Geometry check sheet. Reference: the model listing, model coordinates, mm. Face numbers are marked on the shaded views. Give positions to 0.01 mm unless a question says otherwise; leave off trailing zeros. Order: outer loops, then holes, each group sorted by start corner. A loop starts at its lowest first (then second) coordinate and runs counter-clockwise, first axis right, second up. Notation, with made-up numbers: M -13,-1 L 0,-1 A15 cw 0,10 Z; hole C 80.5,45 d10. An arc over 180 degrees is marked long. Answer as CSV lines item,"result". Start each with the question number.
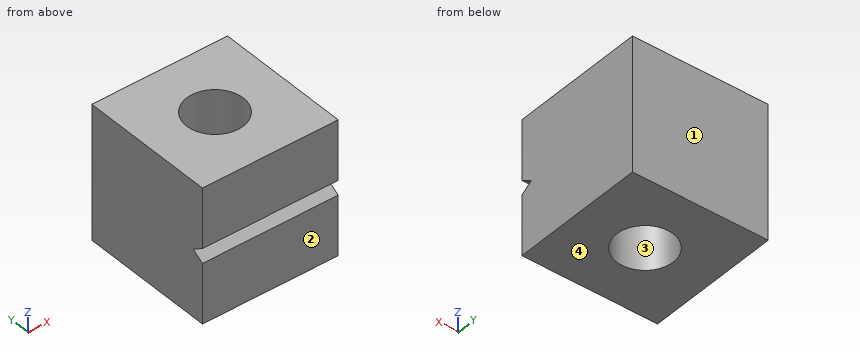
```python
from build123d import *

# Parameters (mm, degrees)
SKETCH1_W               = 19.05
SKETCH1_H               = 19.05
BOSS_EXTRUDE1_DEPTH     = 18.796
SKETCH2_R               = 3.9624
CUT_EXTRUDE1_DEPTH      = 24.124464664
CUT_EXTRUDE2_DEPTH      = 24.124464664
CUT_EXTRUDE2_DEPTH_BACK = 24.124464664


with BuildPart() as part:
    # Sketch1 → Boss-Extrude1 (new body)
    with BuildSketch(Plane.XY):
        Rectangle(SKETCH1_W, SKETCH1_H)
    extrude(amount=BOSS_EXTRUDE1_DEPTH)

    # Sketch2 → Cut-Extrude1 (cut, through all)
    with BuildSketch(Plane.XY.offset(18.796)):
        Circle(SKETCH2_R)
    extrude(amount=-CUT_EXTRUDE1_DEPTH, mode=Mode.SUBTRACT)

    # Sketch3 → Cut-Extrude2 (cut, two sides: drawn at the far end of the back side and taken through both)
    with BuildSketch(Plane(origin=(0, 0, 0), x_dir=(0, 0, -1), z_dir=(1, 0, 0)).offset(-CUT_EXTRUDE2_DEPTH_BACK)):
        Polygon((-39.274452126, -54.498347151), (-10.424511864, -9.525), (-9.398, -7.9248), (-8.371488136, -9.525), (20.478452126, -54.498347151), (20.478452126, -161.361268824), (-39.274452126, -161.361268824), align=None)
    extrude(amount=CUT_EXTRUDE2_DEPTH + CUT_EXTRUDE2_DEPTH_BACK, mode=Mode.SUBTRACT)


solid = part.part
```
Item 1: Scan lines: line 1 along Y through (x, z) = (0, 11.25) (3 decimals); line 2 along Z through (x, y) = (8.75, -8.25); line 3 along X through (y, z) = (1, 6) (3 decimals). Record each from-to range of solid material in increasing order.
Item 2: Draft check along Y on the marked faces 1, 2, 3 and 4. Enter one of: pulls with the +Y half, pulls with the -Y half, needs draft (parallel to the pull), parting line crosses it, or undercut.
Item 3: Section check C-C on z = 12. Record the boundary of the cut face in (x, y) (3 decimals), then the cut area to 3 significant figures.
Item 4: Section check B-B on x = 0. Record the boundary of the cut face in (y, z) (3 decimals).
Item 5: Section check A-A on y = 0. Record the boundary of the cut face in (x, z) (3 decimals).
Numbers:
1,line 1,"-9.525 to -3.962, 3.962 to 9.525"
1,line 2,"0 to 9.19, 9.61 to 18.8"
1,line 3,"-9.525 to -3.834, 3.834 to 9.525"
2,face 1,"pulls with the +Y half"
2,face 2,"pulls with the -Y half"
2,face 3,"undercut"
2,face 4,"needs draft"
3,outline,"M -9.525,-9.525 L 9.525,-9.525 L 9.525,9.525 L -9.525,9.525 Z; hole C 0,0 d7.925"
3,area,"314 mm2"
4,outline,"M -9.525,0 L -3.962,0 L -3.962,18.796 L -9.525,18.796 L -9.525,10.425 L -7.925,9.398 L -9.525,8.371 Z; M 3.962,0 L 9.525,0 L 9.525,18.796 L 3.962,18.796 Z"
5,outline,"M -9.525,0 L -3.962,0 L -3.962,18.796 L -9.525,18.796 Z; M 3.962,0 L 9.525,0 L 9.525,18.796 L 3.962,18.796 Z"
